from build123d import *

# Parameters (mm, degrees)
SALIENTE_EXTRUIR1_DEPTH = 2


with BuildPart() as part:
    # Croquis1 → Saliente-Extruir1 (new body)
    with BuildSketch(Plane(origin=(0, 0, 0), x_dir=(1, 0, 0), z_dir=(0, 1, 0))):
        with BuildLine():
            ThreePointArc((-13.17605398, 4.731976493), (-12.124355653, -7), (-2.490015137, -13.776785714))
            ThreePointArc((-2.490015137, -13.776785714), (0, -16.5), (2.490015137, -13.776785714))
            ThreePointArc((2.490015137, -13.776785714), (12.124355653, -7), (13.17605398, 4.731976493))
            ThreePointArc((13.17605398, 4.731976493), (14.289419162, 8.25), (10.686038843, 9.044809222))
            ThreePointArc((10.686038843, 9.044809222), (0, 14), (-10.686038843, 9.044809222))
            ThreePointArc((-10.686038843, 9.044809222), (-14.289419162, 8.25), (-13.17605398, 4.731976493))
        make_face()
        with BuildLine():
            Line((1.867511353, -10.332589286), (1.333936681, -7.380420918))
            ThreePointArc((1.333936681, -7.380420918), (0, -7.5), (-1.333936681, -7.380420918))
            Line((-1.333936681, -7.380420918), (-1.867511353, -10.332589286))
            ThreePointArc((-1.867511353, -10.332589286), (-10.5, 0), (-1.867511353, 10.332589286))
            Line((-1.867511353, 10.332589286), (-1.333936681, 7.380420918))
            ThreePointArc((-1.333936681, 7.380420918), (0, 7.5), (1.333936681, 7.380420918))
            Line((1.333936681, 7.380420918), (1.867511353, 10.332589286))
            ThreePointArc((1.867511353, 10.332589286), (10.5, 0), (1.867511353, -10.332589286))
        make_face(mode=Mode.SUBTRACT)
    extrude(amount=SALIENTE_EXTRUIR1_DEPTH)


solid = part.part
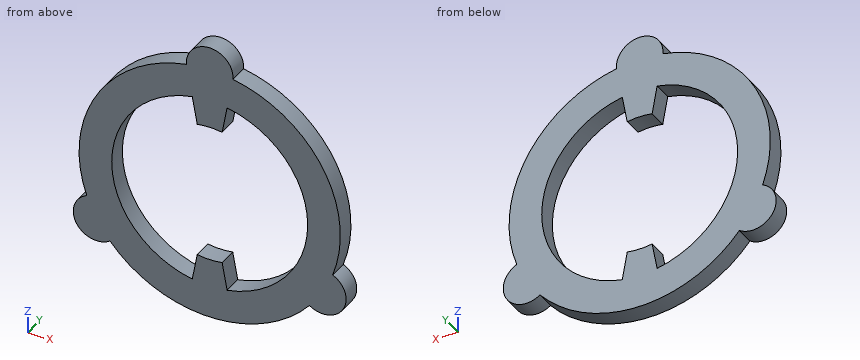
Input: part model. Units: mm. Frame: model coordinates. Give positions to 0.01 mm unless a question says otherwise; leave off trailing zeros. Write each loop counter-clockwise with the first axis right and the second up, starting at its lowest first coordinate (ties: lowest second). Pieces come first, ordered by that corner, then holes. Notation, with made-up numbers: M -33,41 L -23,41 A20 ccw -23,67 Z; hole C 35,49.5 d3. An arc over 180 degrees is marked long. Write item = value, one per line. Start each with the question number.
1) Cut plane D-D on x = -11.25. Return the cut outline in (y, z).
2) Material intervals for line 1 along X through (y, z) = (0.45, 0); line 2 along X through (y, z) = (0.2, -8.5); line 3 along Z through (x, y) = (-8.25, 1.75), sorted ascending. Write a range as [from, to].
3) Cut plane B-B on z = -6. Return the cut outline in (x, y).
4) Cut plane A-A on x = 0. Return the cut outline in (y, z).
5) Cut plane C-C on y = 1.1. Return the cut outline in (x, z).
6) First-contact query: pin 1 Ø1 at (y, z) = (0.5, -4) entering from +X. Flat tip, straight axial feed; report the tip coordinate or a pass-through.
Solved:
q1.outline = M 0,-9.34 L 2,-9.34 L 2,8.33 L 0,8.33 Z
q2.line_1 = [-14, -10.5], [10.5, 14]
q2.line_2 = [-14.12, -6.16], [-1.54, 1.54], [6.16, 14.12]
q2.line_3 = [-11.31, -6.5], [6.5, 11.31]
q3.outline = M -14.42,0 L -8.62,0 L -8.62,2 L -14.42,2 Z; M 8.62,0 L 14.42,0 L 14.42,2 L 8.62,2 Z
q4.outline = M 0,-14 L 2,-14 L 2,-7.5 L 0,-7.5 Z; M 0,7.5 L 2,7.5 L 2,16.5 L 0,16.5 Z
q5.outline = M -13.18,-4.73 A2.5 ccw long -10.69,-9.04 A14 ccw 10.69,-9.04 A2.5 ccw long 13.18,-4.73 A14 ccw 2.49,13.78 A2.5 ccw long -2.49,13.78 A14 ccw Z; hole M -1.87,-10.33 L -1.33,-7.38 A7.5 ccw 1.33,-7.38 L 1.87,-10.33 A10.5 ccw 1.87,10.33 L 1.33,7.38 A7.5 ccw -1.33,7.38 L -1.87,10.33 A10.5 ccw Z
q6.pin_1 = 13.56
